Here's how the part is built. I have some questions about the finished solid (model axes, mm). A direction names the side the tool comes from. Round coordinates to 2 decimals unless told otherwise and drop trailing zeros. Loops run counter-clockwise (first coordinate to the right, second up) from the corner with the lowest first, then second, coordinate; pieces in that order, holes last. Notation, with made-up numbers: M 3.25,-2 L 30.25,-2 A13 cw 30.25,8 Z; hole C -31,80 d9. An arc over 180 degrees is marked long. Answer as a JSON object with one key per item and string values.
from build123d import *

# Parameters (mm, degrees)
SZKIC1_R                    = 5.1
DODANIE_WYCI_GNI_CIE1_DEPTH = 3


with BuildPart() as part:
    # Szkic1 → Dodanie-wyciągnięcie1 (new body)
    with BuildSketch(Plane.XY):
        Polygon((97.5, 0), (-97.5, 0), (-97.5, 35), (-90.283121635, 47.5), (-79.716878365, 47.5), (-72.5, 35), (-72.5, 27.5), (72.5, 27.5), (72.5, 35), (79.716878365, 47.5), (90.283121635, 47.5), (97.5, 35), align=None)
        with Locations((-85, 22)):
            Circle(SZKIC1_R, mode=Mode.SUBTRACT)
        with Locations(Location((85, 22, 0), (0, 0, 180))):
            Circle(SZKIC1_R, mode=Mode.SUBTRACT)
    extrude(amount=DODANIE_WYCI_GNI_CIE1_DEPTH)


solid = part.part
Item 1: For faces 1 (the face through (-93.942, 41.162, 1.479)), 2 (the face through (76.058, 41.162, 1.479)), which set-ups out of +Z, -Z, +X, -X, +Y, -Y let a thin tool reach every point of the face, with its end or its side?
Solution:
{"face 1": "+Z, -Z, -X, +Y", "face 2": "+Z, -Z, +Y"}
Item 2: We'd pull the mould along Y, two halves only. Please class faces 3 (the face through (-90.095, 22.224, 1.479)), 4 (the face through (90.095, 21.776, 1.479)), 5 (the face through (93.84, 41.34, 1.48)), 6 (the face through (1, 19, 0)): +Y half, -Y half, draft (parallel to the pull), parting line (faces both ways), or undercut.
Solution:
{"face 3": "undercut", "face 4": "undercut", "face 5": "+Y half", "face 6": "draft"}
Item 3: I want a section at C-C on y = 22. List the corners of the cut face in (x, z) for me.
Solution:
{"outline": "M -97.5,0 L -90.1,0 L -90.1,3 L -97.5,3 Z; M -79.9,0 L 79.9,0 L 79.9,3 L -79.9,3 Z; M 90.1,0 L 97.5,0 L 97.5,3 L 90.1,3 Z"}
Item 4: I want a section at A-A on y = 33. List the corners of the cut face in (x, z) for me, plus the area to 3 significant figures.
Solution:
{"outline": "M -97.5,0 L -72.5,0 L -72.5,3 L -97.5,3 Z; M 72.5,0 L 97.5,0 L 97.5,3 L 72.5,3 Z", "area": "150 mm2"}
Item 5: If I drill on L1, parallel to X at y = 32.5, z = 1.35; L2, parallel to X at y = 18, z = 1; L3, parallel to X at y = 20, z = 2.9, over which ranges is the centre line in solid material (lowest first)? Write a range as from..to.
Solution:
{"L1": "x = -97.5..-72.5, 72.5..97.5", "L2": "x = -97.5..-88.16, -81.84..81.84, 88.16..97.5", "L3": "x = -97.5..-89.69, -80.31..80.31, 89.69..97.5"}
Item 6: I want a section at B-B on x = 85. List the corners of the cut face in (y, z) for me.
Solution:
{"outline": "M 0,0 L 16.9,0 L 16.9,3 L 0,3 Z; M 27.1,0 L 47.5,0 L 47.5,3 L 27.1,3 Z"}
Item 7: I want a section at D-D on z = 2.35. List the corners of the cut face in (x, y) for me, plus the area to 3 significant figures.
Solution:
{"outline": "M -97.5,0 L 97.5,0 L 97.5,35 L 90.28,47.5 L 79.72,47.5 L 72.5,35 L 72.5,27.5 L -72.5,27.5 L -72.5,35 L -79.72,47.5 L -90.28,47.5 L -97.5,35 Z; hole C -85,22 d10.2; hole C 85,22 d10.2", "area": "6,020 mm2"}
Item 8: For P1, Ø1, axis at x = 0, z = 1.5, coming from the +Y side, with a flat end and sliding along its axis, tell me the tip position at first contact or that it passes through.
Solution:
{"P1": "stops at y = 27.5"}
